```python
from build123d import *

# Parameters (mm, degrees)
F0_R       = 1.4
F0_R_2     = 3.75
F1_DEPTH   = 20
F2_R       = 3.75
F3_DEPTH   = 6
F4_SIZE2   = 5
F4_SIZE    = 1
F4_2_SIZE2 = 5
F4_2_SIZE  = 1
F5_R       = 1.4
F6_DEPTH   = 25
F7_W       = 3
F7_H       = 10
F7_H_2     = 4.4981769323
F7_W_2     = 5.9
F7_H_3     = 5
F8_DEPTH   = 25
F9_DEPTH   = 4


with BuildPart() as f1:
    # F0 (on Top) → F1 (new body)
    with BuildSketch(Plane.XY):
        Polygon((-4.034158995, 3.5947567205), (-24.4, 3.5947567205), (-24.4, -5.2947567205), (-4.034158995, -5.2947567205), (4.034158995, -5.2947567205), (24.4, -5.2947567205), (24.4, 3.5947567205), (4.034158995, 3.5947567205), align=None)
        with Locations((-22, 0)):
            Circle(F0_R, mode=Mode.SUBTRACT)
        with Locations((0, -0.85)):
            Circle(F0_R_2, mode=Mode.SUBTRACT)
        with Locations((22, 0)):
            Circle(F0_R, mode=Mode.SUBTRACT)
    extrude(amount=F1_DEPTH)

    # F2 (on face) → F3 (cut)
    with BuildSketch(Plane.XY.offset(20)):
        with BuildLine():
            ThreePointArc((1.8122189976, -5.2947567205), (3.9836322112, -3.5278114955), (4.8, -0.85))
            ThreePointArc((4.8, -0.85), (3.9836322112, 1.8278114955), (1.8122189976, 3.5947567205))
            Line((1.8122189976, 3.5947567205), (-1.8122189976, 3.5947567205))
            ThreePointArc((-1.8122189976, 3.5947567205), (-4.8, -0.85), (-1.8122189976, -5.2947567205))
            Line((-1.8122189976, -5.2947567205), (1.8122189976, -5.2947567205))
        make_face()
        with Locations((0, -0.85)):
            Circle(F2_R, mode=Mode.SUBTRACT)
        with BuildLine():
            Line((-1.8122189976, 3.5947567205), (1.8122189976, 3.5947567205))
            ThreePointArc((1.8122189976, 3.5947567205), (0, 3.95), (-1.8122189976, 3.5947567205))
        make_face()
        with BuildLine():
            ThreePointArc((-1.8122189976, -5.2947567205), (0, -5.65), (1.8122189976, -5.2947567205))
            Line((1.8122189976, -5.2947567205), (-1.8122189976, -5.2947567205))
        make_face()
    extrude(amount=-F3_DEPTH, mode=Mode.SUBTRACT)

    # F4
    f4_edges = [f1.edges().sort_by_distance(p)[0] for p in [
        (-13.106109, -5.294757, 20),
    ]]
    f4_side = f1.faces().sort_by_distance((-13.89592, -0.879836, 20))[0]
    chamfer(f4_edges, length=F4_SIZE, length2=F4_SIZE2, reference=f4_side)

    # F4#2
    f4_2_edges = [f1.edges().sort_by_distance(p)[0] for p in [
        (13.106109, -5.294757, 20),
    ]]
    f4_2_side = f1.faces().sort_by_distance((13.89592, -0.879836, 20))[0]
    chamfer(f4_2_edges, length=F4_2_SIZE, length2=F4_2_SIZE2, reference=f4_2_side)

    # F5 (on face) → F6 (cut)
    with BuildSketch(Plane(origin=(0, -7.9757276159, 1.5951455232), x_dir=(1, 0, 0), z_dir=(0, -0.9805806757, 0.1961161351))):
        with Locations((-16, 16.9616127755)):
            Circle(F5_R)
        with Locations((16, 16.9616127755)):
            Circle(F5_R)
        with Locations((-16, 8.9616127755)):
            Circle(F5_R)
        with Locations((16, 8.9616127755)):
            Circle(F5_R)
    extrude(amount=-F6_DEPTH, mode=Mode.SUBTRACT)

    # F7 (on face) → F8 (cut)
    with BuildSketch(Plane.XZ.offset(5.2947567205)):
        with Locations((-20, 9)):
            Rectangle(F7_W, F7_H)
        with Locations((-4, 6.2490884662)):
            Rectangle(F7_W, F7_H_2)
        with Locations((4, 6.2490884662)):
            Rectangle(F7_W, F7_H_2)
        with Locations((12, 9)):
            Rectangle(F7_W, F7_H)
        with Locations((20, 9)):
            Rectangle(F7_W, F7_H)
        Polygon((-21.5, 4), (-21.5, 14), (-18.5, 14), (-18.5, 15), (-24.4, 15), (-24.4, 4), align=None)
        with Locations((-21.45, 17.5)):
            Rectangle(F7_W_2, F7_H_3)
        with Locations((21.45, 17.5)):
            Rectangle(F7_W_2, F7_H_3)
        Polygon((21.5, 4), (24.4, 4), (24.4, 15), (18.5, 15), (18.5, 14), (21.5, 14), align=None)
        with Locations((-12, 9)):
            Rectangle(F7_W, F7_H)
    extrude(amount=-F8_DEPTH, mode=Mode.SUBTRACT)

    # F0 (on Top) → F9 (join)
    with BuildSketch(Plane.XY):
        with BuildLine():
            Line((4.034158995, -5.2947567205), (-4.034158995, -5.2947567205))
            ThreePointArc((-4.034158995, -5.2947567205), (0, -6.8525245607), (4.034158995, -5.2947567205))
        make_face()
        with BuildLine():
            ThreePointArc((4.034158995, 3.5947567205), (0, 5.1525245607), (-4.034158995, 3.5947567205))
            Line((-4.034158995, 3.5947567205), (4.034158995, 3.5947567205))
        make_face()
    extrude(amount=F9_DEPTH)


solid = f1.part
```
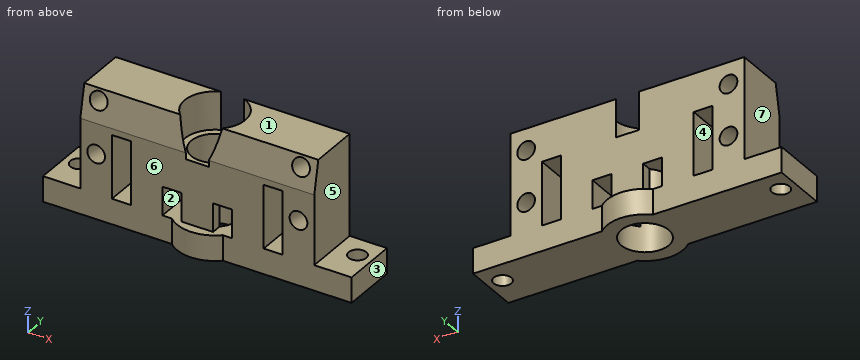
The model under review builds one solid part; all positions refer to its coordinate system, in mm. Face numbers are marked on the shaded views. A direction names the side the tool comes from. Coordinates: 2 decimals unless noted, no trailing zeros. Order: outer loops, then holes, each group sorted by start corner. A loop starts at its lowest first (then second) coordinate and runs counter-clockwise, first axis right, second up. Notation, with made-up numbers: M -30.5,31.25 L 4.5,31.25 A17 cw 4.5,53.25 Z; hole C 56,-20.5 d7. An arc over 180 degrees is marked long. One line per question, with ' | ' between items.
(1) Machinability: for the marked faces 4, 5, 6 and 7, which of the approach directions +Z, -Z, +X, -X, +Y, -Y give a long, thin tool a straight path to every point of the face, cutting with its end or side? Answer none if there is none.
Geometry results:
face 4: +Y, -Y | face 5: +Z, +X, +Y, -Y | face 6: +Z, -Y | face 7: +Z, -X, +Y, -Y
(2) Add section C-C, the plane x = 0. Write out the cut boundary in (y, z).
Geometry results:
outline: M -6.85,0 L -4.6,0 L -4.6,14 L -5.29,14 L -5.29,4 L -6.85,4 Z; M 2.9,0 L 5.15,0 L 5.15,4 L 3.59,4 L 3.59,14 L 2.9,14 Z
(3) Add section A-A, the plane x = -22. Write out the cut boundary in (y, z), then the cut area to 3 significant figures.
Geometry results:
outline: M -5.29,0 L -1.4,0 L -1.4,4 L -5.29,4 Z; M 1.4,0 L 3.59,0 L 3.59,4 L 1.4,4 Z | area: 24.4 mm²
(4) For probe 1 along X at (y, z) = (3, 4.75); probe 2 along Y at (x, z) = (-22, 1.4); probe 3 along X at (y, z) = (-0.85, 4.5), list the stretches that pass through material, from the lowest coordinate up. Write a range as from..to.
Geometry results:
probe 1: x = -18.5..-13.5, -10.5..-5.5, -2.5..2.5, 5.5..10.5, 13.5..18.5 | probe 2: y = -5.29..-1.4, 1.4..3.59 | probe 3: x = -18.5..-13.5, -10.5..-5.5, 5.5..10.5, 13.5..18.5
(5) Add section B-B, the plane y = -2.75. State how many separate pieces and enclosed holes the cut face has, then the cut area to 3 significant figures.
Geometry results:
separate pieces: 2 | enclosed holes: 6 | area: 538 mm²
(6) The part is to be moulded in two halves that separate along X. For the marked faces 1, 2 and 3, say which applies: +X half, -X half, draft (parallel to the pull), parting line (faces both ways), or undercut.
Geometry results:
face 1: draft | face 2: undercut | face 3: +X half
(7) Insertion check: pin 1 (3 mm diameter, centred on y = 3.5, z = 12, fed in from -X); pin 2 (4.5 mm diameter, centred on y = -2.5, z = 9.5, fed in from +X); pin 3 (3.5 mm diameter, centred on x = -0.5, y = 0, fed in from +Z); pin 4 (4.5 mm diameter, centred on x = 22, y = 0, fed in from +Z). Each pin has a flat end and moves straight along its axis. Give the tip position at first contact, or say it passes through.
Geometry results:
pin 1: stops at x = -18.5 | pin 2: stops at x = 18.5 | pin 3: passes through | pin 4: stops at z = 4
